```python
from build123d import *

# Parameters (mm, degrees)
F3_R      = 8
F3_R_2    = 6
F4_DEPTH  = 50
F5_R      = 11
F5_R_2    = 9.2
F6_DEPTH  = 50
F7_R      = 9.2
F8_DEPTH  = 57.7284067103
F9_R      = 29.9655409023
F10_DEPTH = 12.5


with BuildPart() as f4:
    # F3 (on 3pt) → F4 (new body)
    with BuildSketch(Plane(origin=(0, 0, 0), x_dir=(0.9659258263, 0, -0.2588190451), z_dir=(-0.2588190451, 0, -0.9659258263))):
        Circle(F3_R)
        Circle(F3_R_2, mode=Mode.SUBTRACT)
    extrude(amount=-F4_DEPTH)

    # F5 (on Right) → F6 (join)
    with BuildSketch(Plane.YZ):
        with Locations((0, 50)):
            Circle(F5_R)
        with Locations((0, 50)):
            Circle(F5_R_2, mode=Mode.SUBTRACT)
    extrude(amount=F6_DEPTH)

    # F7 (on face) → F8 (cut, through all)
    with BuildSketch(Plane.YZ.offset(50)):
        with Locations((0, 50)):
            Circle(F7_R)
    extrude(amount=-F8_DEPTH, mode=Mode.SUBTRACT)

    # F9 (on Front) → F10 (cut, symmetric)
    with BuildSketch(Plane.XZ):
        with Locations((51.6765899956, 31.8527929485)):
            Circle(F9_R)
    extrude(amount=F10_DEPTH, both=True, mode=Mode.SUBTRACT)


solid = f4.part
```
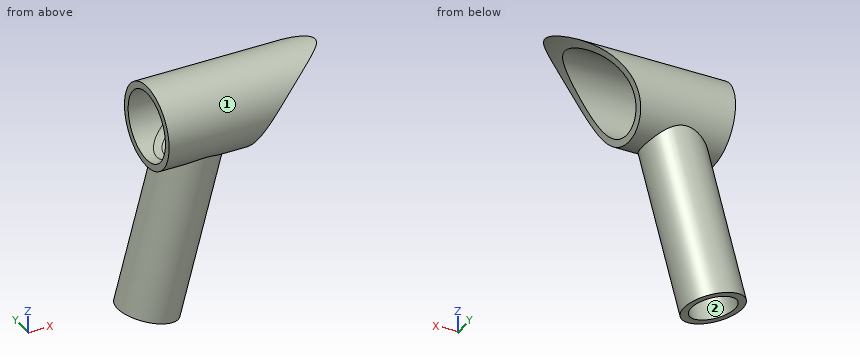
Geometry: final body of the model. Coordinates: model frame, mm. Face numbers are marked on the shaded views. Give positions to 0.01 mm unless a question says otherwise; leave off trailing zeros. Loops run counter-clockwise (first coordinate to the right, second up) from the corner with the lowest first, then second, coordinate; pieces in that order, holes last. Notation, with made-up numbers: (65, 86.25) -> (71, 86.25) arc R28 cw to (71, 117.25) -> close; hole circle Ø6 at (-17.75, -5.5). An arc over 180 degrees is marked (long way). Return JSON: item names as keys, results as strings.
Item 1: Mould query, pull axis Y, two halves, no side actions, for the marked faces 1 and 2. Classes: released by +Y, released by -Y, zero draft, split by the parting line, or undercut.
Filled in:
{"face 1": "split by the parting line", "face 2": "undercut"}
Item 2: Line query: line 1 (Y direction, x = 25, z = 50); line 2 (Z direction, x = 20, y = 0); line 3 (X direction, y = -4.5, z = 5.5). Output: solid intervals per line, ascending.
Filled in:
{"line 1": "-11 to -9.2, 9.2 to 11", "line 2": "39 to 40.8, 59.2 to 61", "line 3": "-5.37 to -2.63, 5.58 to 8.32"}
Item 3: Section B-B, the plane y = 0. Output: boundary loops of the cut face in (x, z).
Filled in:
{"outline": "(-7.73, 2.07) -> (-5.8, 1.55) -> (4.24, 39) -> (16.66, 39) -> (5.8, -1.55) -> (7.73, -2.07) -> (18.73, 39) -> (22.58, 39) arc R29.97 cw to (23.08, 40.8) -> (0, 40.8) -> (0, 39) -> (2.17, 39) -> close; (0, 59.2) -> (39.43, 59.2) arc R29.97 cw to (44.72, 61) -> (0, 61) -> close"}
Item 4: Pin query (flat end, axial travel): P1, Ø5, axis at y = -5.5, z = 4.5, coming from the +X side; P2, Ø12, axis at y = -4.5, z = 21.5, coming from the -X side; P3, Ø3, axis at x = 37, y = 0.5, coming from the -Z side. Return the tip coordinate at first contact, or that it passes through.
Filled in:
{"P1": "x = 9.07", "P2": "x = -3.77", "P3": "z = 58.98"}
Item 5: Section C-C, the plane x = 38.5. Output: boundary loops of the cut face in (y, z).
Filled in:
{"outline": "(-6.65, 58.77) -> (-2.79, 58.77) arc R9.2 cw to (2.79, 58.77) -> (6.65, 58.77) arc R11 ccw to start"}
Item 6: Section D-D, the plane x = 12.5. Count the separate pieces of the cut face and the enclosed holes in it, plus the area to 3 significant figures.
Filled in:
{"separate pieces": "1", "enclosed holes": "2", "area": "263 mm^2"}
Item 7: Section A-A, the plane z = 50. Output: boundary loops of the cut face in (x, y), plus the area to 3 significant figures.
Filled in:
{"outline": "(0, -11) -> (27.83, -11) -> (27.83, -9.2) -> (0, -9.2) -> close; (0, 9.2) -> (27.83, 9.2) -> (27.83, 11) -> (0, 11) -> close", "area": "100 mm^2"}
